from build123d import *

# Parameters (mm, degrees)
SKETCH1_R           = 9.398
SKETCH1_R_2         = 34.589431616
BOSS_EXTRUDE1_DEPTH = 3.175
FILLET1_R           = 25.4
CUT_EXTRUDE1_DEPTH  = 7.35


with BuildPart() as part:
    # Sketch1 → Boss-Extrude1 (new body, symmetric)
    with BuildSketch(Plane(origin=(-101.6, 0, 0), x_dir=(0, 0, -1), z_dir=(1, 0, 0))):
        with BuildLine():
            Line((181.785515067, 280.321615274), (242.984426747, 222.593234225))
            Line((242.984426747, 222.593234225), (254.108513166, 138.043359025))
            ThreePointArc((254.108513166, 138.043359025), (264.972075139, 127.118097295), (278.378708009, 134.710232547))
            Line((278.378708009, 134.710232547), (317.047217946, 225.215098942))
            ThreePointArc((317.047217946, 225.215098942), (315.782704, 260.070612955), (288.110795268, 281.301988787))
            Line((288.110795268, 281.301988787), (193.202213869, 301.969191763))
            ThreePointArc((193.202213869, 301.969191763), (179.266512438, 295.48442041), (181.785515067, 280.321615274))
        make_face()
        with Locations((190.5, 289.56)):
            Circle(SKETCH1_R, mode=Mode.SUBTRACT)
        with Locations((279.4, 241.3)):
            Circle(SKETCH1_R_2, mode=Mode.SUBTRACT)
        with Locations((266.7, 139.7)):
            Circle(SKETCH1_R, mode=Mode.SUBTRACT)
    extrude(amount=BOSS_EXTRUDE1_DEPTH, both=True)

    # Fillet1
    fillet1_edges = [part.edges().sort_by_distance(p)[0] for p in [
        (-101.6, 222.593234225, -242.984426747),
    ]]
    fillet(fillet1_edges, radius=FILLET1_R)

    # Sketch2 → Cut-Extrude1 (cut, through all)
    with BuildSketch(Plane(origin=(-98.425, 0, 0), x_dir=(0, 0, -1), z_dir=(1, 0, 0))):
        with BuildLine():
            Line((196.625780281, 275.052266892), (238.924841277, 235.151944416))
            ThreePointArc((238.924841277, 235.151944416), (244.181424008, 262.17316378), (265.361199141, 279.757107685))
            Line((265.361199141, 279.757107685), (205.932122543, 292.698327232))
            ThreePointArc((205.932122543, 292.698327232), (204.429524577, 282.213718691), (196.625780281, 275.052266892))
        make_face()
        with BuildLine():
            Line((250.779296509, 212.027275618), (258.524425256, 153.159549829))
            ThreePointArc((258.524425256, 153.159549829), (268.842626828, 155.301559354), (278.201366063, 150.45723397))
            Line((278.201366063, 150.45723397), (302.603477212, 207.571144307))
            ThreePointArc((302.603477212, 207.571144307), (275.892741569, 200.511077492), (250.779296509, 212.027275618))
        make_face()
    extrude(amount=-CUT_EXTRUDE1_DEPTH, mode=Mode.SUBTRACT)


solid = part.part
Input: part model. Units: mm. Frame: model coordinates. A direction names the side the tool comes from. Round coordinates to 2 decimals unless told otherwise and drop trailing zeros. Order: outer loops, then holes, each group sorted by start corner. A loop starts at its lowest first (then second) coordinate and runs counter-clockwise, first axis right, second up. Notation, with made-up numbers: (50, -17) - (95, -17) arc R11 ccw to (95, 4) - close; hole circle Ø8 at (77, 30). An arc over 180 degrees is marked (long way). Use a Markdown table: item, result.
1. First-contact query: pin 1 (1.5 mm diameter, centred on x = -102.5, y = 197, fed in from +Z); pin 2 (1.5 mm diameter, centred on x = -100, y = 277.5, fed in from -Z); pin 3 (8 mm diameter, centred on y = 167.5, z = -242.5, fed in from -X). Flat tips, straight axial feed; report the tip coordinate or a pass-through.
Evaluation:
| item | result |
|---|---|
| pin 1 | z = -246.25 |
| pin 2 | z = -299.88 |
| pin 3 | through |
2. Section B-B on y = 239. Return the cut outline in (x, z) (3 decimals).
Evaluation:
| item | result |
|---|---|
| outline | (-104.775, -320.275) - (-98.425, -320.275) - (-98.425, -313.913) - (-104.775, -313.913) - close; (-104.775, -244.887) - (-98.425, -244.887) - (-98.425, -238.525) - (-104.775, -238.525) - close; (-104.775, -234.845) - (-98.425, -234.845) - (-98.425, -225.591) - (-104.775, -225.591) - close |
3. Section D-D on y = 216.5. Return the cut outline in (x, z) (3 decimals), then the cut area to 3 significant figures.
Evaluation:
| item | result |
|---|---|
| outline | (-104.775, -313.324) - (-98.425, -313.324) - (-98.425, -303.512) - (-104.775, -303.512) - close; (-104.775, -255.288) - (-98.425, -255.288) - (-98.425, -243.617) - (-104.775, -243.617) - close |
| area | 136 mm^2 |
4. Section A-A on z = -224. Return the cut outline in (x, y) (3 decimals).
Evaluation:
| item | result |
|---|---|
| outline | (-104.775, 240.501) - (-98.425, 240.501) - (-98.425, 249.23) - (-104.775, 249.23) - close; (-104.775, 288.764) - (-98.425, 288.764) - (-98.425, 295.263) - (-104.775, 295.263) - close |
5. Mould query, pull axis Y, two halves, no side actions, for faces 1 (the face through (-101.64, 136.1, -275.38)), 2 (the face through (-101.56, 259.62, -316.01)), 3 (the face through (-101.556, 127.152, -264.743)). Classes: +Y half, -Y half, draft (parallel to the pull), parting line (faces both ways), or undercut.
Evaluation:
| item | result |
|---|---|
| face 1 | undercut |
| face 2 | parting line |
| face 3 | -Y half |
6. Access query for faces 4 (the face through (-101.556, 286.137, -236.063)), 5 (the face through (-101.56, 221.99, -241.54)). Directions: +Z, -Z, +X, -X, +Y, -Y. A direction counts if a zero-diameter tool reaches every point of the face in a straight line with its end or side. Return the directions, or none.
Evaluation:
| item | result |
|---|---|
| face 4 | +X, -X |
| face 5 | +Z, +X, -X, -Y |
7. Material intervals for probe 1 along Y at (x, z) = (-101.5, -270); probe 2 along Z at (x, y) = (-99.25, 204); probe 3 along Y at (x, z) = (-100, -267), sorted ascending.
Evaluation:
| item | result |
|---|---|
| probe 1 | 127.44 to 130.9, 148.5 to 155.1, 201.45 to 208.01, 274.59 to 285.25 |
| probe 2 | -307.98 to -301.08, -296.27 to -262.53, -251.84 to -245.43 |
| probe 3 | 127 to 130.31, 149.09 to 155.45, 202.28 to 209.01, 273.59 to 285.9 |
8. Section C-C on x = -101.25. Return the cut outline in (y, z).
Evaluation:
| item | result |
|---|---|
| outline | (134.71, -278.38) - (225.22, -317.05) arc R40.94 ccw to (281.3, -288.11) - (301.97, -193.2) arc R12.7 ccw to (280.32, -181.79) - (228.8, -236.41) arc R25.4 cw to (213.63, -244.16) - (138.04, -254.11) arc R12.7 ccw to start; hole circle Ø18.8 at (139.7, -266.7); hole (150.46, -278.2) - (207.57, -302.6) arc R40.94 cw to (212.03, -250.78) - (153.16, -258.52) arc R15.75 cw to start; hole circle Ø69.18 at (241.3, -279.4); hole (235.15, -238.92) arc R40.94 cw to (279.76, -265.36) - (292.7, -205.93) arc R15.75 cw to (275.05, -196.63) - close; hole circle Ø18.8 at (289.56, -190.5) |
